Input: part model. Units: mm. Frame: model coordinates. Give positions to 0.01 mm unless a question says otherwise; leave off trailing zeros. Order: outer loops, then holes, each group sorted by start corner. A loop starts at its lowest first (then second) coordinate and runs counter-clockwise, first axis right, second up.
```python
from build123d import *

# Parameters (mm, degrees)
F0_R     = 0.5
F1_DEPTH = 2
F2_R     = 3


with BuildPart() as f1:
    # F0 (on Top) → F1 (new body)
    with BuildSketch(Plane.XY):
        Polygon((-11.8603997611, -5.284095183), (2.8522056527, -5.284095183), (2.8522056527, 6.8704825826), (-17.2913148999, 19.4052960724), (-35.9591057258, 6.2361949424), align=None)
        Circle(F0_R, mode=Mode.SUBTRACT)
        with Locations((-28.9777747887, 7.7645713531)):
            Circle(F0_R, mode=Mode.SUBTRACT)
        with Locations((-16.7303260748, 14.8356391649)):
            Circle(F0_R, mode=Mode.SUBTRACT)
        with Locations((-13.5, 8)):
            Circle(F0_R, mode=Mode.SUBTRACT)
        with Locations((-8.5, 8)):
            Circle(F0_R, mode=Mode.SUBTRACT)
    extrude(amount=F1_DEPTH)

    # F2
    f2_edges = [f1.edges().sort_by_distance(p)[0] for p in [
        (-17.291315, 19.405296, 1),
        (2.852206, -5.284095, 1),
        (2.852206, 6.870483, 1),
        (-35.959106, 6.236195, 1),
        (-11.8604, -5.284095, 1),
    ]]
    fillet(f2_edges, radius=F2_R)


solid = f1.part
```
1) Line query: probe 1 along X at (y, z) = (7.75, 1.5); probe 2 along Y at (x, z) = (-13.5, 0.3); probe 3 along Y at (x, z) = (-29, 1.9). Output: solid intervals per line, ascending.
2) Cut plane B-B (z = 1.2). Return the cut outline in (x, y).
3) Cut plane C-C (y = 0). Return the cut outline in (x, z), then the cut area to 3 significant figures.
4) Pull-direction query (Y, two-part tool) for faces 1 (the face through (-25.257, 13.786, 0.986)), 2 (the face through (-15, 7, 2)), 3 (the face through (-14, 8, 1)); classes: pulls with the +Y half, pulls with the -Y half, needs draft (parallel to the pull), parting line crosses it, or undercut.
5) Cut plane A-A (x = -13.5). Return the cut outline in (y, z), then the cut area to 3 significant figures.
6) Cut plane D-D (y = 10.5). Return the cut outline in (x, z), then the cut area to 3 significant figures.
Geometry says:
1. probe 1: x = -32.87 to -29.48, -28.48 to -13.93, -13.07 to -8.93, -8.07 to 1.44
1. probe 2: y = -4.5 to 7.5, 8.5 to 17.05
1. probe 3: y = 2.91 to 7.27, 8.26 to 11.15
2. outline: (-31.78, 9.19) arc R3 ccw to (-31.34, 4.03) - (-12.47, -4.99) arc R3 ccw to (-11.18, -5.28) - (-0.15, -5.28) arc R3 ccw to (2.85, -2.28) - (2.85, 5.2) arc R3 ccw to (1.44, 7.75) - (-15.6, 18.35) arc R3 ccw to (-18.92, 18.26) - close; hole circle Ø1 at (-28.98, 7.76); hole circle Ø1 at (-16.73, 14.84); hole circle Ø1 at (-13.5, 8); hole circle Ø1 at (-8.5, 8); hole circle Ø1 at (0, 0)
3. outline: (-22.91, 0) - (-0.5, 0) - (-0.5, 2) - (-22.91, 2) - close; (0.5, 0) - (2.85, 0) - (2.85, 2) - (0.5, 2) - close
3. area: 49.5 mm2
4. face 1: pulls with the +Y half
4. face 2: needs draft
4. face 3: undercut
5. outline: (-4.5, 0) - (7.5, 0) - (7.5, 2) - (-4.5, 2) - close; (8.5, 0) - (17.05, 0) - (17.05, 2) - (8.5, 2) - close
5. area: 41.1 mm2
6. outline: (-29.91, 0) - (-2.98, 0) - (-2.98, 2) - (-29.91, 2) - close
6. area: 53.9 mm2
